from build123d import *

# Parameters (mm, degrees)
SKETCH_W     = 67
SKETCH_H     = 155
SKETCH_R     = 1.5
SKETCH_R_2   = 2.5
PAD_DEPTH    = 10
SKETCH001_W  = 50
SKETCH001_H  = 50
POCKET_DEPTH = 5


with BuildPart() as part:
    # Sketch → Pad (new body)
    with BuildSketch(Plane.YZ):
        Rectangle(SKETCH_W, SKETCH_H)
        with Locations((-15.5, 14.5)):
            Circle(SKETCH_R, mode=Mode.SUBTRACT)
        with Locations((15.5, 14.5)):
            Circle(SKETCH_R, mode=Mode.SUBTRACT)
        with Locations((15.5, -16.5)):
            Circle(SKETCH_R, mode=Mode.SUBTRACT)
        with Locations((-15.5, -16.5)):
            Circle(SKETCH_R, mode=Mode.SUBTRACT)
        with Locations((24.5, 52.5)):
            Circle(SKETCH_R_2, mode=Mode.SUBTRACT)
        with Locations((-24.5, 52.5)):
            Circle(SKETCH_R_2, mode=Mode.SUBTRACT)
        with Locations((14, 68)):
            Circle(SKETCH_R, mode=Mode.SUBTRACT)
        with Locations((-14, 68)):
            Circle(SKETCH_R, mode=Mode.SUBTRACT)
        with BuildLine():
            ThreePointArc((-9.5, -13.694169), (0, -23.194169), (9.5, -13.694169))
            Line((9.5, -13.694169), (9.5, 14.305831))
            ThreePointArc((9.5, 14.305831), (0, 23.805831), (-9.5, 14.305831))
            Line((-9.5, -13.694169), (-9.5, 14.305831))
        make_face(mode=Mode.SUBTRACT)
    extrude(amount=PAD_DEPTH)

    # Sketch001 (on Face18 of Pad) → Pocket (cut)
    with BuildSketch(Plane.YZ.offset(10)):
        Rectangle(SKETCH001_W, SKETCH001_H)
    extrude(amount=-POCKET_DEPTH, mode=Mode.SUBTRACT)


solid = part.part
Source: CAD feature listing. Evaluate the final solid. Frame: model axes, mm. A direction names the side the tool comes from. Coordinates: 2 decimals unless noted, no trailing zeros. Write each loop counter-clockwise with the first axis right and the second up, starting at its lowest first coordinate (ties: lowest second). Pieces come first, ordered by that corner, then holes. Notation, with made-up numbers: M 86.5,22 L 99.5,22 A15 ccw 99.5,35 Z; hole C 48.25,15.25 d5. An arc over 180 degrees is marked long. Use a Markdown table: item, result.
1) Section B-B, the plane z = 68. Output: boundary loops of the cut face in (x, y), then the cut area to 3 significant figures.
Conclusion:
| item | result |
|---|---|
| outline | M 0,-33.5 L 10,-33.5 L 10,-15.5 L 0,-15.5 Z; M 0,-12.5 L 10,-12.5 L 10,12.5 L 0,12.5 Z; M 0,15.5 L 10,15.5 L 10,33.5 L 0,33.5 Z |
| area | 610 mm^2 |
2) Mould query, pull axis Z, two halves, no side actions, for faces 1 (the cylindrical face through (4.93, -14.195, 69.487)), 2 (the flat face through (5, 0, 77.5)), 3 (the flat face through (5, 0, -77.5)). Classes: pulls with the +Z half, pulls with the -Z half, needs draft (parallel to the pull), parting line crosses it, or undercut.
Conclusion:
| item | result |
|---|---|
| face 1 | undercut |
| face 2 | pulls with the +Z half |
| face 3 | pulls with the -Z half |
3) Section C-C, the plane z = 3.5. Output: boundary loops of the cut face in (x, y).
Conclusion:
| item | result |
|---|---|
| outline | M 0,-33.5 L 10,-33.5 L 10,-25 L 5,-25 L 5,-9.5 L 0,-9.5 Z; M 0,9.5 L 5,9.5 L 5,25 L 10,25 L 10,33.5 L 0,33.5 Z |
4) Ray query, L1, parallel to Z at x = 6.5, y = -8.5; L2, parallel to Z at x = 7.5, y = 14; L3, parallel to Y at x = 4.75, z = 8. Return the intervals inside material, ascending.
Conclusion:
| item | result |
|---|---|
| L1 | z = -77.5 to -25, 25 to 77.5 |
| L2 | z = -77.5 to -25, 25 to 66.5, 69.5 to 77.5 |
| L3 | y = -33.5 to -9.5, 9.5 to 33.5 |
5) Reachability of faces 4 (the flat face through (10, 29, 1)), 5 (the flat face through (8, 0, 25)), 6 (the flat face through (2, -9.5, 0)) from +Z, -Z, +X, -X, +Y, -Y: full face, straight path, thin tool, end or side. Return the list, or none.
Conclusion:
| item | result |
|---|---|
| face 4 | +Z, -Z, +X, +Y, -Y |
| face 5 | +X |
| face 6 | +X, -X |
6) Section D-D, the plane y = -19.5. Output: boundary loops of the cut face in (x, z), then the cut area to 3 significant figures.
Conclusion:
| item | result |
|---|---|
| outline | M 0,-77.5 L 10,-77.5 L 10,-25 L 5,-25 L 5,25 L 10,25 L 10,77.5 L 0,77.5 Z |
| area | 1,300 mm^2 |
7) First-contact query: pin 1 Ø25 at (y, z) = (0, 3) entering from +X. Flat tip, straight axial feed; report the tip coordinate or a pass-through.
Conclusion:
| item | result |
|---|---|
| pin 1 | stops at x = 5 |
8) Section A-A, the plane y = 0. Output: boundary loops of the cut face in (x, z).
Conclusion:
| item | result |
|---|---|
| outline | M 0,-77.5 L 10,-77.5 L 10,-25 L 5,-25 L 5,-23.19 L 0,-23.19 Z; M 0,23.81 L 5,23.81 L 5,25 L 10,25 L 10,77.5 L 0,77.5 Z |
